Design review of the part built by this model. Coordinates are the model's own, in mm. Coordinates: 2 decimals unless noted, no trailing zeros. Write each loop counter-clockwise with the first axis right and the second up, starting at its lowest first coordinate (ties: lowest second). Pieces come first, ordered by that corner, then holes.
Q1. For pin 1 Ø3 at (x, z) = (-33.5, 1) entering from -Y; pin 2 Ø1.5 at (y, z) = (-50.5, 2.5) entering from +X; pin 3 Ø3 at (y, z) = (-53, 4) entering from +X, all flat-tipped, find the tip position at first contact; note any pin that passes through.
Q2. Take a section at C-C, the plane y = -34. Write out the cut boundary in (x, z).
Q3. Take a section at A-A, the plane z = 0.95. State how many separate pieces and enclosed holes the cut face has, plus the area to 3 significant figures.
Q4. For L1, parallel to Y at x = 0, z = 2.7; L2, parallel to X at y = -61, z = 1.4; L3, parallel to X at y = -45.5, z = 1.8, list the stretches that pass through material, from the lowest coordinate up.
Q5. Take a section at B-B, the plane x = -52. Write out the cut boundary in (y, z).
from build123d import *

# Parameters (mm, degrees)
F1_DEPTH = 5
F2_R     = 1.5
F3_DEPTH = 25


# Not quite as in the source:
# - a feature names something its author has since deleted; it is built from what else it names


with BuildPart() as f1:
    # F0 (on Top) → F1 (new body)
    with BuildSketch(Plane.XY):
        with BuildLine():
            ThreePointArc((-97.4828772247, 0), (-67.2370800722, -63.7098067384), (-2.5426874445, -91.7879705417))
            Line((-2.5426874445, -91.7879705417), (7.5769329952, -91.7879705417))
            ThreePointArc((7.5769329952, -91.7879705417), (72.2713256229, -63.7098067384), (102.5171227753, 0))
            Line((102.5171227753, 0), (102.5171227753, 50.5402684212))
            Line((102.5171227753, 50.5402684212), (-97.4828772247, 50.5402684212))
            Line((-97.4828772247, 50.5402684212), (-97.4828772247, 0))
        make_face()
    extrude(amount=F1_DEPTH)

    # F2 (on face) → F3 (cut)
    with BuildSketch(Plane.XY.offset(5)):
        with Locations((-72.3256510152, -23.5000285577)):
            Circle(F2_R)
        with Locations((-61.4798521783, -43.0486559433)):
            Circle(F2_R)
        with Locations((-42.6908970166, -60.9689194803)):
            Circle(F2_R)
        with Locations((-19.2692746164, -71.9139118934)):
            Circle(F2_R)
        with Locations((0, -74.8913536115)):
            Circle(F2_R)
        with Locations((19.5851995713, -73.0929598765)):
            Circle(F2_R)
        with Locations((44.2583380034, -63.2074572013)):
            Circle(F2_R)
        with Locations((64.7310261921, -45.3251524957)):
            Circle(F2_R)
        with Locations((76.7870070898, -24.9496110183)):
            Circle(F2_R)
        with Locations((0, 14.4641017541)):
            Circle(F2_R)
    extrude(amount=-F3_DEPTH, mode=Mode.SUBTRACT)


solid = f1.part
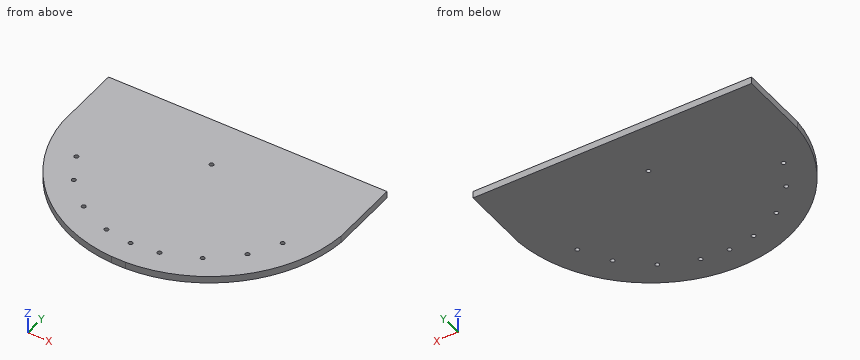
Responses:
1. pin 1: stops at y = -85.79
1. pin 2: stops at x = 84.28
1. pin 3: stops at x = 83.01
2. outline: (-88.42, 0) - (93.46, 0) - (93.46, 5) - (-88.42, 5) - close
3. separate pieces: 1
3. enclosed holes: 10
3. area: 24,200 mm2
4. L1: y = -91.79 to -76.39, -73.39 to 12.96, 15.96 to 50.54
4. L2: x = -69.94 to -44.19, -41.19 to 74.97
4. L3: x = -82.11 to 63.24, 66.22 to 87.14
5. outline: (-75.82, 0) - (50.54, 0) - (50.54, 5) - (-75.82, 5) - close
